Autodesk Inventor part; units mm, degrees
ref_plane "YZ Plane" through (0, 0, 0) normal (1, 0, 0) x (0, 1, 0)
ref_plane "XZ Plane" through (0, 0, 0) normal (0, 1, 0) x (-1, 0, 0)
ref_plane "XY Plane" through (0, 0, 0) normal (0, 0, 1) x (1, 0, 0)
sketch "Sketch1" plane through (0, 0, 0) normal (0, 0, 1) x (1, 0, 0)
  line L0 (0, 0) -> (2000, 0)
  line L1 (2000, 0) -> (2000, 200)
  line L2 (2000, 200) -> (0, 200)
  line L3 (0, 200) -> (0, 0)
  dimension "d0" = 2000
  dimension "d1" = 200
extrude "Extrusion1" add sketch "Sketch1" along normal blind 25.4
sketch "Sketch2" plane through (0, 0, 25.4) normal (0, 0, 1) x (1, 0, 0)
  circle A0 centre (1893.2025, 100) radius 62.8623
  point P0 (0, 0)
  dimension "d4" = 125.7246
  dimension "d5" = 1895.8417
extrude "Extrusion2" add sketch "Sketch2" along normal blind 127
properties part number "Belt"
The listing builds one solid part. Answer for the finished solid, in the listing's coordinates (mm). A direction names the side the tool comes from. Coordinates: 2 decimals unless noted, no trailing zeros. Write each loop counter-clockwise with the first axis right and the second up, starting at its lowest first coordinate (ties: lowest second). Pieces come first, ordered by that corner, then holes. Notation, with made-up numbers: M 66.25,39 L 85.25,39 A19 cw 85.25,69 Z; hole C -31,-24.75 d1. An arc over 180 degrees is marked long. Use a Markdown table: item, result. Add a question column.
1. Section C-C (z = 48) is taken. Give the vertices of the cut face in (x, y).
2. Section B-B (x = 517) is taken. Give the vertices of the cut face in (y, z), plus the area to 3 significant figures.
3. Which of the six approach directions +Z, -Z, +X, -X, +Y, -Y give full straight-line access (tool end or side, diameter ignored) to faces 1 (the cylindrical face through (1953.162, 81.118, 88.011)), 2 (the flat face through (1892, 101, 152.4))?
4. Straight lines are drawn through the part: line 1 along Z through (x, y) = (1423.5, 178); line 2 along X through (y, z) = (154, 129); line 3 along X through (y, z) = (133, 115.5). For each, find the intervals that lie inside material, in ascending order. Write a range as [from, to].
5. Section A-A (y = 100) is taken. Give the vertices of the cut face in (x, z), plus the area to 3 significant figures.
6. Section D-D (y = 19.5) is taken. Give the vertices of the cut face in (x, z).
7. Given P1, Ø6, axis at y = 162, z = 26, coming from the +X side; P2, Ø4, axis at x = 846.5, y = 148, coming from the +Z side; P3, Ø2, axis at y = 104.5, z = 43.5, coming from the +X side, each flat-ended and moving along its own axis, determine where each tip first touches the part or whether it passes through.
Data:
| question | item | result |
|---|---|---|
| 1 | outline | C 1893.2,100 d125.72 |
| 2 | outline | M 0,0 L 200,0 L 200,25.4 L 0,25.4 Z |
| 2 | area | 5,080 mm2 |
| 3 | face 1 | +Z |
| 3 | face 2 | +Z, +X, -X, +Y, -Y |
| 4 | line 1 | z = [0, 25.4] |
| 4 | line 2 | x = [1861.02, 1925.38] |
| 4 | line 3 | x = [1839.7, 1946.71] |
| 5 | outline | M 0,0 L 2000,0 L 2000,25.4 L 1956.06,25.4 L 1956.06,152.4 L 1830.34,152.4 L 1830.34,25.4 L 0,25.4 Z |
| 5 | area | 66,800 mm2 |
| 6 | outline | M 0,0 L 2000,0 L 2000,25.4 L 0,25.4 Z |
| 7 | P1 | stops at x = 2000 |
| 7 | P2 | stops at z = 25.4 |
| 7 | P3 | stops at x = 1955.97 |
